Source: CAD feature listing. Evaluate the final solid. Frame: model axes, mm. Face numbers are marked on the shaded views. A direction names the side the tool comes from. Round coordinates to 2 decimals unless told otherwise and drop trailing zeros. Order: outer loops, then holes, each group sorted by start corner. A loop starts at its lowest first (then second) coordinate and runs counter-clockwise, first axis right, second up. Notation, with made-up numbers: M -18,-7 L -6,-7 A33 cw -6,25 Z; hole C -39,2.25 d7. An arc over 180 degrees is marked long. Answer in a Markdown table with one row per item. Add a question column.
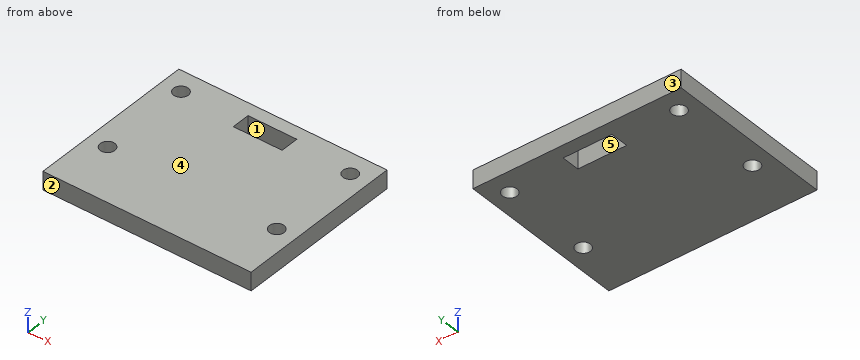
```python
from build123d import *

# Parameters (mm, degrees)
SKETCH1_W               = 45.5
SKETCH1_H               = 37
SKETCH1_W_2             = 10.66
SKETCH1_H_2             = 4
BOSS_EXTRUDE1_DEPTH     = 4
SKETCH3_R               = 1.6
CUT_EXTRUDE5_DEPTH      = 10
CUT_EXTRUDE5_DEPTH_BACK = 1


with BuildPart() as part:
    # Sketch1 → Boss-Extrude1 (new body)
    with BuildSketch(Plane.XY):
        with Locations((22.75, 18.5)):
            Rectangle(SKETCH1_W, SKETCH1_H)
        with Locations((22.75, 32.14)):
            Rectangle(SKETCH1_W_2, SKETCH1_H_2, mode=Mode.SUBTRACT)
    extrude(amount=BOSS_EXTRUDE1_DEPTH)

    # Sketch3 → Cut-Extrude5 (cut, two sides)
    with BuildSketch(Plane.XY) as cut_extrude5_sk:
        with Locations((41.27584891, 32.252592082)):
            Circle(SKETCH3_R)
        with Locations((41.27584891, 12.252592082)):
            Circle(SKETCH3_R)
        with Locations((4.27584891, 12.252592082)):
            Circle(SKETCH3_R)
        with Locations((4.27584891, 32.252592082)):
            Circle(SKETCH3_R)
    extrude(amount=CUT_EXTRUDE5_DEPTH, mode=Mode.SUBTRACT)
    extrude(cut_extrude5_sk.sketch, amount=-CUT_EXTRUDE5_DEPTH_BACK, mode=Mode.SUBTRACT)


solid = part.part
```
(1) Draft query along Y for the marked faces 1, 2 and 3. Return one class per face: +Y half, -Y half, draft (parallel to the pull), parting line (faces both ways), or undercut.
(2) Cut plane A-A (x = 20.5). Return loops of the section in (y, z).
(3) Line query: line 1 (Y direction, x = 18, z = 3.3); line 2 (Y direction, x = 40, z = 3.3); line 3 (X direction, y = 13.5, z = 2.6). Output: solid intervals per line, ascending. Write a range as from..to.
(4) Cut plane B-B (z = 1.5). Return loops of the section in (x, y), and give its area (3 significant figures).
(5) Access query for the marked faces 4 and 5. Directions: +Z, -Z, +X, -X, +Y, -Y. A direction counts if a zero-diameter tool reaches every point of the face in a straight line with its end or side. Return the directions, or none.
Answer list:
| question | item | result |
|---|---|---|
| 1 | face 1 | undercut |
| 1 | face 2 | -Y half |
| 1 | face 3 | +Y half |
| 2 | outline | M 0,0 L 30.14,0 L 30.14,4 L 0,4 Z; M 34.14,0 L 37,0 L 37,4 L 34.14,4 Z |
| 3 | line 1 | 0..30.14, 34.14..37 |
| 3 | line 2 | 0..11.29, 13.22..31.29, 33.22..37 |
| 3 | line 3 | 0..3.27, 5.28..40.27, 42.28..45.5 |
| 4 | outline | M 0,0 L 45.5,0 L 45.5,37 L 0,37 Z; hole C 4.28,12.25 d3.2; hole C 4.28,32.25 d3.2; hole M 17.42,30.14 L 28.08,30.14 L 28.08,34.14 L 17.42,34.14 Z; hole C 41.28,12.25 d3.2; hole C 41.28,32.25 d3.2 |
| 4 | area | 1,610 mm² |
| 5 | face 4 | +Z, +X, -X, +Y, -Y |
| 5 | face 5 | +Z, -Z |
